Answer from the drawing. Dimensions are ordinates in mm from the lowest x, y and z of the part. A direction names the side the tool comes from. Round coordinates to 2 decimals unless told otherwise and drop trailing zeros. Write each loop counter-clockwise with the first axis right and the second up, starting at its lowest first coordinate (ties: lowest second). Pieces come first, ordered by that corner, then holes.
1. Determine the mould class of the marked faces 1, 2, 3 and 4 for opening direction X: pulls with the +X half, pulls with the -X half, needs draft (parallel to the pull), parting line crosses it, or undercut.
2. Find section B-B (x = 42.5). Write down the section's boundary in (y, z) (1 decimal).
3. A tool of negligible diameter and unlimited length cuts with its end or side. For the marked faces 5, 6, 7, 8 and 9, from which of +Z, -Z, +X, -X, +Y, -Y can it reach the whole face along a straight path? Write none if from no direction.
4. Flat-ended cylindrical pins translate along their axes: pin 1 Ø6.5 at (x, z) = (48, 15.5) entering from -Y; pin 2 Ø8 at (x, y) = (72, 12) entering from -Z (1 decimal); pin 3 Ø5 at (x, y) = (41.5, 52.5) entering from +Z (1 decimal); pin 4 Ø6 at (y, z) = (75.5, 17) entering from +X. Find the tip coordinate at first contact, or state that the pin passes through.
5. Find section D-D (y = 67.5). Write down the section's boundary in (x, z) (1 decimal).
6. Find section A-A (z = 16.5). Write down the section's boundary in (x, y).
7. Straight lines are drawn through the part: probe 1 along Y at (x, z) = (28.5, 9); probe 2 along Y at (x, z) = (76.5, 34.5) (1 decimal); probe 3 along X at (y, z) = (70.5, 33.5) (1 decimal). For each, find the intervals that lie inside material, in ascending order.
8. Find section C-C (z = 37). Write down the section's boundary in (x, y) (1 decimal), and give its area (3 significant figures).
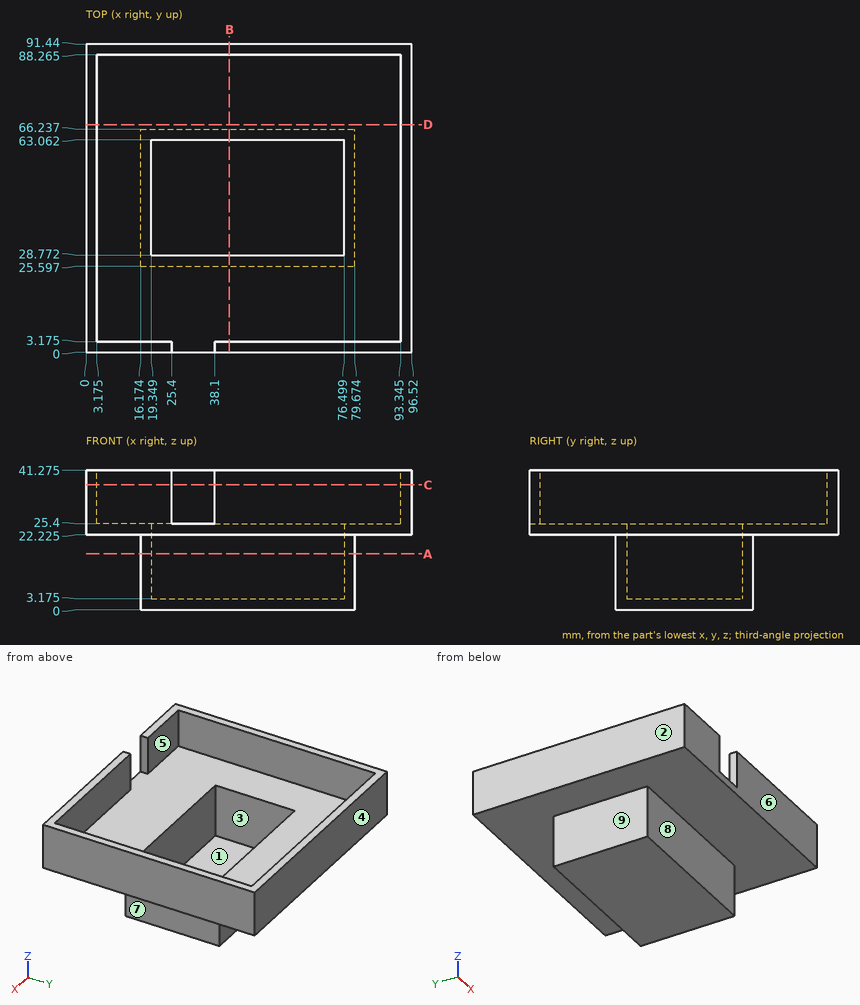
Worked answers:
1. face 1: undercut
1. face 2: pulls with the -X half
1. face 3: undercut
1. face 4: needs draft
2. outline: (0, 22.2) - (25.6, 22.2) - (25.6, 0) - (66.2, 0) - (66.2, 22.2) - (91.4, 22.2) - (91.4, 41.3) - (88.3, 41.3) - (88.3, 25.4) - (63.1, 25.4) - (63.1, 3.2) - (28.8, 3.2) - (28.8, 25.4) - (3.2, 25.4) - (3.2, 41.3) - (0, 41.3) - close
3. face 5: +Z
3. face 6: +Z, -Z, +X, -X, -Y
3. face 7: -Z, +X, +Y, -Y
3. face 8: -Z, +X, -X, -Y
3. face 9: -Z, -X, +Y, -Y
4. pin 1: stops at y = 25.6
4. pin 2: stops at z = 22.2
4. pin 3: stops at z = 3.2
4. pin 4: passes through
5. outline: (0, 22.2) - (96.5, 22.2) - (96.5, 41.3) - (93.3, 41.3) - (93.3, 25.4) - (3.2, 25.4) - (3.2, 41.3) - (0, 41.3) - close
6. outline: (16.17, 25.6) - (79.67, 25.6) - (79.67, 66.24) - (16.17, 66.24) - close; hole (19.35, 28.77) - (76.5, 28.77) - (76.5, 63.06) - (19.35, 63.06) - close
7. probe 1: y = 25.6 to 28.77, 63.06 to 66.24
7. probe 2: y = 0 to 3.2, 88.3 to 91.4
7. probe 3: x = 0 to 3.2, 93.3 to 96.5
8. outline: (0, 0) - (25.4, 0) - (25.4, 3.2) - (3.2, 3.2) - (3.2, 88.3) - (93.3, 88.3) - (93.3, 3.2) - (38.1, 3.2) - (38.1, 0) - (96.5, 0) - (96.5, 91.4) - (0, 91.4) - close
8. area: 1,110 mm2
